Read the model definition and answer for the solid it produces. Units are mm, in the model's axes. A direction names the side the tool comes from. Give positions to 0.01 mm unless a question says otherwise; leave off trailing zeros. Loops run counter-clockwise (first coordinate to the right, second up) from the corner with the lowest first, then second, coordinate; pieces in that order, holes last. Notation, with made-up numbers: (69.25, 28.5) - (108.25, 28.5) arc R10 ccw to (108.25, 43.5) - close; hole circle Ø4 at (33, 85.5). An arc over 180 degrees is marked (long way). Use a Markdown table: item, result. Add a question column.
Item 1: A cutting plane is placed at D-D (y = -4). Determine the outline of the cut face in (x, z).
Item 2: A cutting plane is placed at B-B (z = 0). Determine the outline of the cut face in (x, y), plus the area to 3 significant figures.
Item 3: A cutting plane is placed at A-A (x = 0). Determine the outline of the cut face in (y, z).
Item 4: A cutting plane is placed at C-C (y = 17). Determine the outline of the cut face in (x, z), plus the area to 3 significant figures.
Item 5: Each of these flat-tipped pins is pushed along its axis until it touches: P1, Ø2, axis at y = -3, z = 13.5, coming from the +X side; P2, Ø8, axis at y = -15.5, z = 10.5, coming from the -X side; P3, Ø2, axis at x = 8, y = 3, coming from the +Z side; P4, Ø8, axis at x = -0.5, y = -7.5, coming from the -Z side. Where does it stop, or does it pass through?
Item 6: Which of the six approach directions +Z, -Z, +X, -X, +Y, -Y give full straight-line access (tool end or side, diameter ignored) to faces 1 (the face through (0, -20, 0)), 2 (the face through (-13, 0, 5))?
Item 7: Consider probe 1 along Y at (x, z) = (4, -13); probe 2 along X at (y, z) = (16, 0); probe 3 along Y at (x, z) = (-10, 3). Determine where each line is inside the solid, lowest interval first. Write a range as [from, to].
Autodesk Inventor part; units mm, degrees
ref_plane "YZ Plane" through (0, 0, 0) normal (1, 0, 0) x (0, 1, 0)
ref_plane "XZ Plane" through (0, 0, 0) normal (0, 1, 0) x (-1, 0, 0)
ref_plane "XY Plane" through (0, 0, 0) normal (0, 0, 1) x (1, 0, 0)
sketch "Sketch1" plane through (0, 0, 0) normal (0, 0, 1) x (1, 0, 0)
  line L0 (0, 0) -> (0, 20)
  line L1 (0, 20) -> (13.45, 20)
  line L2 (13.45, 20) -> (13.45, 13.2)
  line L3 (0, 0) -> (13.45, 0)
  line L4 (13.45, 0) -> (13.45, 5.2)
  arc A0 (13.45, 13.2) -> (13.45, 5.2) centre (13.45, 9.2) ccw
  dimension "d0" = 20
  dimension "d1" = 13.45
  dimension "d2" = 6.8
  dimension "d3" = 13.45
  dimension "d4" = 8
  dimension "d5" = 4
revolve "Revolution1" add sketch "Sketch1" angle 360 about axis through (0, 0, 0) along (0, 1, 0)
chamfer "Chamfer1" distance 0.2 angle 45 1 edges at (-13.45, 20, 0)
sketch "Sketch2" plane through (0, 0, 0) normal (0, -1, 0) x (1, 0, 0)
  circle A0 centre (0, 0) radius 13.45
  circle A1 centre (0, 0) radius 17
  dimension "d10" = 34
extrude "Extrusion1" add sketch "Sketch2" along normal blind 20 contours A0 | A1
chamfer "Chamfer2" distance 0.2 angle 45 1 edges at (-17, 0, 0)
properties part number "slik_clamp_head38_stud"
Geometry says:
| question | item | result |
|---|---|---|
| 1 | outline | circle Ø34 at (0, 0) |
| 2 | outline | (-17, -20) - (17, -20) - (17, -0.2) - (16.8, 0) - (13.45, 0) - (13.45, 5.2) arc R4 cw to (13.45, 13.2) - (13.45, 19.8) - (13.25, 20) - (-13.25, 20) - (-13.45, 19.8) - (-13.45, 13.2) arc R4 cw to (-13.45, 5.2) - (-13.45, 0) - (-16.8, 0) - (-17, -0.2) - close |
| 2 | area | 1,170 mm² |
| 3 | outline | (-20, -17) - (-0.2, -17) - (0, -16.8) - (0, -13.45) - (5.2, -13.45) arc R4 cw to (13.2, -13.45) - (19.8, -13.45) - (20, -13.25) - (20, 13.25) - (19.8, 13.45) - (13.2, 13.45) arc R4 cw to (5.2, 13.45) - (0, 13.45) - (0, 16.8) - (-0.2, 17) - (-20, 17) - close |
| 4 | outline | circle Ø26.9 at (0, 0) |
| 4 | area | 568 mm² |
| 5 | P1 | x = 11.52 |
| 5 | P2 | x = -15.71 |
| 5 | P3 | z = 11.48 |
| 5 | P4 | z = -17 |
| 6 | face 1 | +Z, -Z, +X, -X, -Y |
| 6 | face 2 | +Y |
| 7 | probe 1 | [-20, 0] |
| 7 | probe 2 | [-13.45, 13.45] |
| 7 | probe 3 | [-20, 6.57], [11.83, 20] |
